For this review, use the dimensioned drawing (mm, ordinates from the lowest corner) and the shaded views. A direction names the side the tool comes from. Give positions to 0.01 mm unless a question says otherwise; leave off trailing zeros. Loops run counter-clockwise (first coordinate to the right, second up) from the corner with the lowest first, then second, coordinate; pieces in that order, holes last. Notation, with made-up numbers: (42.5, 56) -> (74.5, 56) arc R24 ccw to (74.5, 74) -> close; hole circle Ø5 at (-36.75, 9.25). An arc over 180 degrees is marked (long way). Use a Markdown table: item, result. Add a question column.
1. Add section D-D (z = 1.5). State the section outline as (x, y) points, and give its area (3 significant figures).
2. Draft analysis for pull direction Y (two halves, no side actions). For the marked faces 1, 2, 3 and 4, state which applies: pulls with the +Y half, pulls with the -Y half, needs draft (parallel to the pull), parting line crosses it, or undercut.
3. Add section A-A (y = 11). State the section outline as (x, z) points, and give its area (3 significant figures).
4. Add section C-C (z = 5). State the section outline as (x, y) points.
5. Add section B-B (x = 8). State the section outline as (y, z) points.
6. For the marked faces 5, 6 and 7, list the 3-axis set-ups (+Z, -Z, +X, -X, +Y, -Y) from which the entire face can be reached by the end or side of a thin tool; tool diameter is ignored.
7. To check wall thickness, follow line 1 (Y direction, x = 8, z = 1.55); line 2 (Z direction, x = 9, y = 26); line 3 (Y direction, x = 11.5, z = 2.25). State the ranges of each line that lie inside material, in increasing order.
8. For pin 1 Ø1 at (x, y) = (6, 18) entering from +Z; pin 2 Ø1.6 at (x, y) = (8, 1.5) entering from -Z, all flat-tipped, find the tip position at first contact; note any pin that passes through.
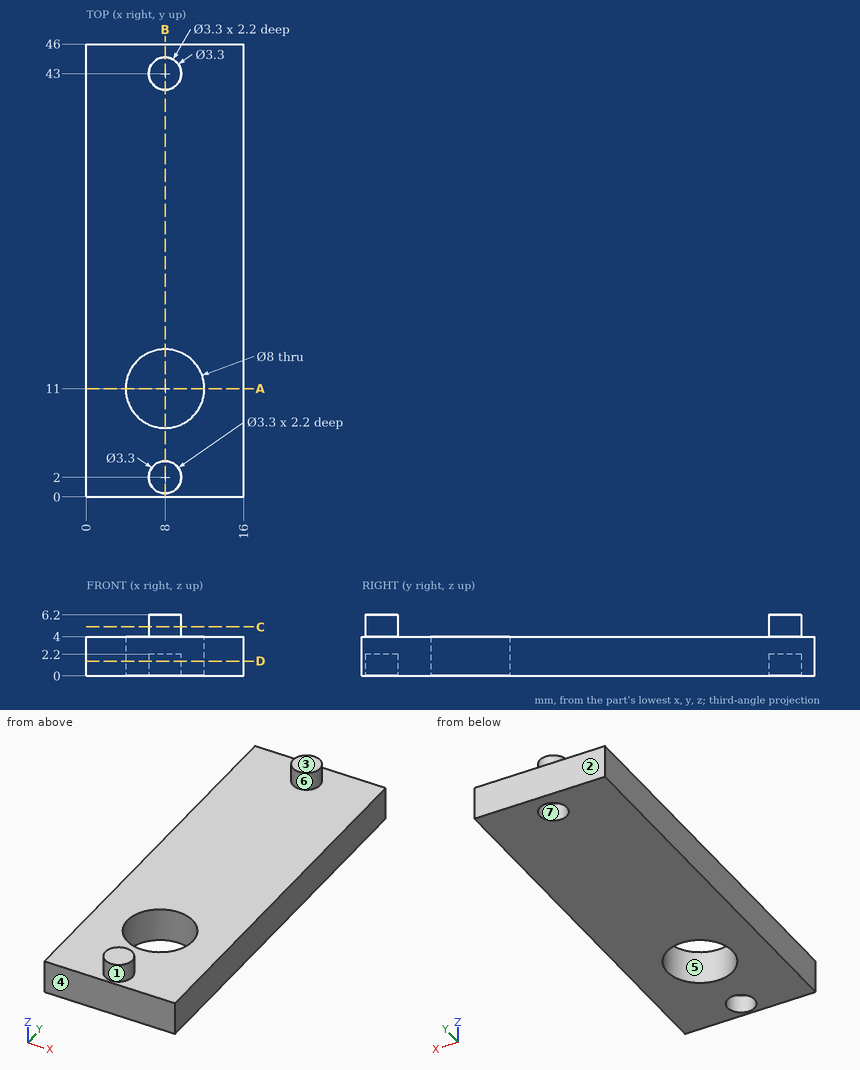
Taken from the geometry:
| question | item | result |
|---|---|---|
| 1 | outline | (0, 0) -> (16, 0) -> (16, 46) -> (0, 46) -> close; hole circle Ø8 at (8, 11); hole circle Ø3.3 at (8, 2); hole circle Ø3.3 at (8, 43) |
| 1 | area | 669 mm^2 |
| 2 | face 1 | undercut |
| 2 | face 2 | pulls with the +Y half |
| 2 | face 3 | needs draft |
| 2 | face 4 | pulls with the -Y half |
| 3 | outline | (0, 0) -> (4, 0) -> (4, 4) -> (0, 4) -> close; (12, 0) -> (16, 0) -> (16, 4) -> (12, 4) -> close |
| 3 | area | 32.0 mm^2 |
| 4 | outline | circle Ø3.3 at (8, 2); circle Ø3.3 at (8, 43) |
| 5 | outline | (0, 0) -> (0.35, 0) -> (0.35, 2.2) -> (3.65, 2.2) -> (3.65, 0) -> (7, 0) -> (7, 4) -> (3.65, 4) -> (3.65, 6.2) -> (0.35, 6.2) -> (0.35, 4) -> (0, 4) -> close; (15, 0) -> (41.35, 0) -> (41.35, 2.2) -> (44.65, 2.2) -> (44.65, 0) -> (46, 0) -> (46, 4) -> (44.65, 4) -> (44.65, 6.2) -> (41.35, 6.2) -> (41.35, 4) -> (15, 4) -> close |
| 6 | face 5 | +Z, -Z |
| 6 | face 6 | +Z |
| 6 | face 7 | -Z |
| 7 | line 1 | y = 0 to 0.35, 3.65 to 7, 15 to 41.35, 44.65 to 46 |
| 7 | line 2 | z = 0 to 4 |
| 7 | line 3 | y = 0 to 9.06, 12.94 to 46 |
| 8 | pin 1 | stops at z = 4 |
| 8 | pin 2 | stops at z = 2.2 |
